```python
from build123d import *

# Parameters (mm, degrees)
BOSS_EXTRUDE1_DEPTH = 8
SKETCH2_R           = 1.5
CUT_EXTRUDE1_DEPTH  = 6
SKETCH3_R           = 1.5
BOSS_EXTRUDE2_DEPTH = 6


with BuildPart() as part:
    # Sketch1 → Boss-Extrude1 (new body)
    with BuildSketch(Plane(origin=(0, 0, 0), x_dir=(1, 0, 0), z_dir=(0, 1, 0))):
        Polygon((2.213376496, -2.195669484), (3.0081938, 0.819005532), (0.794817304, 3.014675016), (-2.213376496, 2.195669484), (-3.0081938, -0.819005532), (-0.794817304, -3.014675016), align=None)
    extrude(amount=BOSS_EXTRUDE1_DEPTH)

    # Sketch2 → Cut-Extrude1 (cut)
    with BuildSketch(Plane(origin=(0, 8, 0), x_dir=(1, 0, 0), z_dir=(0, 1, 0))):
        Circle(SKETCH2_R)
    extrude(amount=-CUT_EXTRUDE1_DEPTH, mode=Mode.SUBTRACT)

    # Sketch3 → Boss-Extrude2 (add)
    with BuildSketch(Plane.XZ):
        Circle(SKETCH3_R)
    extrude(amount=BOSS_EXTRUDE2_DEPTH)


solid = part.part
```
Geometry check sheet. Reference: the model listing, model coordinates, mm. A direction names the side the tool comes from. Coordinates: 2 decimals unless noted, no trailing zeros. Order: outer loops, then holes, each group sorted by start corner. A loop starts at its lowest first (then second) coordinate and runs counter-clockwise, first axis right, second up. Notation, with made-up numbers: M 34.25,36 L 58.25,36 A27 ccw 58.25,68 Z; hole C 11.5,-17.75 d11. An arc over 180 degrees is marked long. One line per question, with ' | ' between items. Start each with the question number.
Item 1: Draft check along X on faces 3 (the flat face through (-1.4, 0, -1.4)), 4 (the cylindrical face through (-1.5, 5.04, -0.07)), 5 (the flat face through (2.605, 3.944, 0.709)), 6 (the flat face through (0, 2, 0)). Enter one of: pulls with the +X half, pulls with the -X half, needs draft (parallel to the pull), parting line crosses it, or undercut.
Item 2: Set-up check for faces 1 (the cylindrical face through (-1.5, -2.96, 0.07)), 2 (the flat face through (-1.4, 8, -1.4)): record each of +Z, -Z, +X, -X, +Y, -Y from which the full face is reachable in a straight line by a thin tool's end or side.
Item 3: Gauge pin test, flat ends, axial feed: pin 1 (1.5 mm diameter, centred on x = 0, z = 0, fed in from +Y); pin 2 (1 mm diameter, centred on x = -0.5, y = 6, fed in from -Z); pin 3 (1 mm diameter, centred on y = 4, z = 2, fed in from +X). Record the tip position at first contact, or that the pin passes through.
Item 4: Cross-section at A-A on y = 5.25. Enter the section's corners in (x, z).
Item 5: Cross-section at C-C on y = 1.75. Enter the section's corners in (x, z), then the cut area to 3 significant figures.
Item 6: Material ranges on L1, parallel to Z at x = 0, y = 6.65; L2, parallel to X at y = 6.5, z = 0; L3, parallel to Z at x = -0.5, y = 3.5, recorded low to high. Write a range as [from, to].
Item 7: Cross-section at B-B on x = 1. Enter the section's corners in (y, z).
Item 8: Cross-section at D-D on z = 0. Enter the section's corners in (x, y), then the cut area to 3 significant figures.
Findings:
1) face 3: needs draft | face 4: undercut | face 5: pulls with the +X half | face 6: undercut
2) face 1: -Y | face 2: +Z, -Z, +X, -X, +Y
3) pin 1: stops at y = 2 | pin 2: stops at z = -2.8 | pin 3: stops at x = 2.4
4) outline: M -3.01,0.82 L -2.21,-2.2 L 0.79,-3.01 L 3.01,-0.82 L 2.21,2.2 L -0.79,3.01 Z; hole C 0,0 d3
5) outline: M -3.01,0.82 L -2.21,-2.2 L 0.79,-3.01 L 3.01,-0.82 L 2.21,2.2 L -0.79,3.01 Z | area: 25.3 mm²
6) L1: z = [-2.8, -1.5], [1.5, 2.8] | L2: x = [-2.79, -1.5], [1.5, 2.79] | L3: z = [-2.66, -1.41], [1.41, 2.93]
7) outline: M -6,-1.12 L 0,-1.12 L 0,-2.81 L 8,-2.81 L 8,-1.12 L 2,-1.12 L 2,1.12 L 8,1.12 L 8,2.53 L 0,2.53 L 0,1.12 L -6,1.12 Z
8) outline: M -2.79,0 L -1.5,0 L -1.5,-6 L 1.5,-6 L 1.5,0 L 2.79,0 L 2.79,8 L 1.5,8 L 1.5,2 L -1.5,2 L -1.5,8 L -2.79,8 Z | area: 44.7 mm²
